Part print with two shaded views. Sizes in mm from the minimum x, y, z corner. Give positions to 0.01 mm unless a question says otherwise; leave off trailing zeros. Order: outer loops, then holes, each group sorted by start corner. A loop starts at its lowest first (then second) coordinate and runs counter-clockwise, first axis right, second up. Notation, with made-up numbers: M -21,59.5 L -13,59.5 A23 cw -13,96.5 Z; hole C -4.5,31 d10. An arc over 180 degrees is marked long. Answer as CSV lines item,"result".
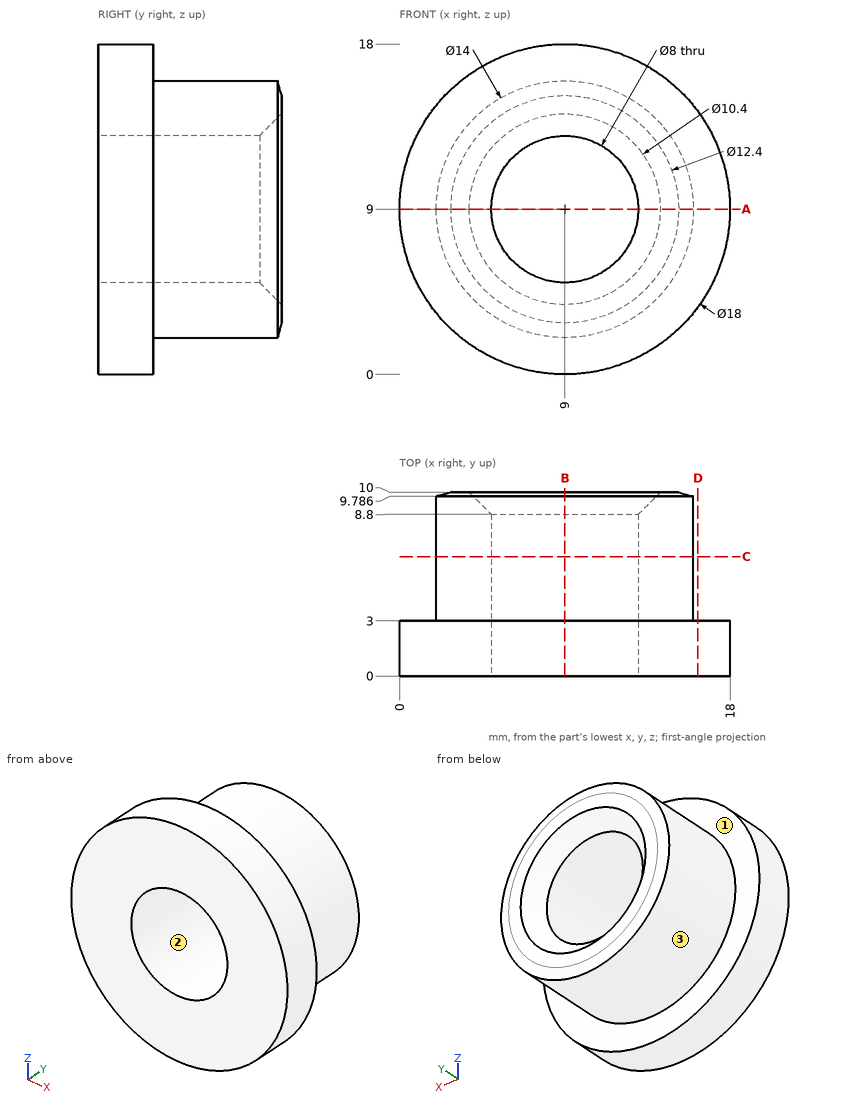
Item 1: Pull direction X, two halves, no side cores. Call the marked faces 1, 2 and 3: released by +X, released by -X, zero draft, split by the parting line, or undercut.
Geometry says:
face 1,"zero draft"
face 2,"undercut"
face 3,"split by the parting line"
Item 2: Band-saw the part on C-C (y = 6.5). Give the cut face in (x, z).
Geometry says:
outline,"C 9,9 d14; hole C 9,9 d8"
Item 3: Band-saw the part on D-D (x = 16.25). Give the cut face in (y, z).
Geometry says:
outline,"M 0,3.67 L 3,3.67 L 3,14.33 L 0,14.33 Z"
Item 4: Band-saw the part on A-A (z = 9). Give the cut face in (x, y) (1 decimal).
Geometry says:
outline,"M 0,0 L 5,0 L 5,8.8 L 3.8,10 L 2.8,10 L 2,9.8 L 2,3 L 0,3 Z; M 13,0 L 18,0 L 18,3 L 16,3 L 16,9.8 L 15.2,10 L 14.2,10 L 13,8.8 Z"
Item 5: Probe line 1 along Z through (x, y) = (9, 4.25); line 2 along Z through (x, y) = (9, 2); line 3 along Y through (x, z) = (4.5, 16.75). List the from-to ranges inside material, lowest first. Write a range as from..to.
Geometry says:
line 1,"z = 2..5, 13..16"
line 2,"z = 0..5, 13..18"
line 3,"y = 0..3"
Item 6: Band-saw the part on B-B (x = 9). Give the cut face in (y, z) (1 decimal).
Geometry says:
outline,"M 0,0 L 3,0 L 3,2 L 9.8,2 L 10,2.8 L 10,3.8 L 8.8,5 L 0,5 Z; M 0,13 L 8.8,13 L 10,14.2 L 10,15.2 L 9.8,16 L 3,16 L 3,18 L 0,18 Z"
Item 7: Drop flat-ended pins along their axis: pin 1 (1.5 mm diameter, centred on y = 4.5, z = 4, fed in from +X); pin 2 (6 mm diameter, centred on x = 10.5, z = 9.5, fed in from +Y); pin 3 (4 mm diameter, centred on x = 14, y = 5.5, fed in from +Z) (1 decimal). Give the stop position or say it passes through.
Geometry says:
pin 1,"stops at x = 14.56"
pin 2,"stops at y = 9.38"
pin 3,"stops at z = 15.3"
